Model file for the job. Use its own axes, mm. A direction names the side the tool comes from. Round coordinates to 2 decimals unless told otherwise and drop trailing zeros. Order: outer loops, then holes, each group sorted by start corner. A loop starts at its lowest first (then second) coordinate and runs counter-clockwise, first axis right, second up. Notation, with made-up numbers: (88, -14.5) -> (138, -14.5) arc R16 cw to (138, -4.5) -> close; hole circle Ø4 at (54, 32). An arc over 180 degrees is marked (long way). Use CSV: the item, a comma, the result in double quotes.
```python
from build123d import *

# Parameters (mm, degrees)
F1_DEPTH = 5


with BuildPart() as f1:
    # F0 (on Top) → F1 (new body)
    with BuildSketch(Plane.XY):
        with BuildLine():
            Line((-4.36566, 79.626773), (-32.035204, 75.337673))
            Line((-32.035204, 75.337673), (-22.550609, 14.151324))
            Line((-22.550609, 14.151324), (-13.305154, 10.567361))
            ThreePointArc((-13.305154, 10.567361), (-11.394923, 13.178449), (-8.43507, 14.484602))
            ThreePointArc((-8.43507, 14.484602), (-3.410814, 13.054214), (-1.227681, 8.308365))
            ThreePointArc((-1.227681, 8.308365), (-1.334221, 7.159279), (-1.650209, 6.049369))
            ThreePointArc((-1.650209, 6.049369), (-3.56044, 3.438281), (-6.520293, 2.132127))
            Line((-6.520293, 2.132127), (-5.001368, -7.666653))
            Line((-5.001368, -7.666653), (52.729861, -30.045928))
            Line((52.729861, -30.045928), (62.850163, -3.938851))
            Line((62.850163, -3.938851), (5.118934, 18.440424))
            Line((5.118934, 18.440424), (-4.36566, 79.626773))
        make_face()
        with BuildLine():
            Line((-13.305154, 10.567361), (-22.550609, 14.151324))
            Line((-22.550609, 14.151324), (-70.797245, -24.65575))
            Line((-70.797245, -24.65575), (-53.248003, -46.473727))
            Line((-53.248003, -46.473727), (-5.001368, -7.666653))
            Line((-5.001368, -7.666653), (-6.520293, 2.132127))
            ThreePointArc((-6.520293, 2.132127), (-12.347765, 4.391123), (-13.305154, 10.567361))
        make_face()
    extrude(amount=F1_DEPTH)


solid = f1.part
```
Q1. Cut at B-B (y = -18.5). Give the cut face in (x, z), plus the area to 3 significant figures.
From the geometry:
outline,"(-63.14, 0) -> (-18.47, 0) -> (-18.47, 5) -> (-63.14, 5) -> close; (22.95, 0) -> (57.21, 0) -> (57.21, 5) -> (22.95, 5) -> close"
area,"395 mm²"
Q2. Cut at D-D (y = 49.5). Give the cut face in (x, z), plus the area to 3 significant figures.
From the geometry:
outline,"(-28.03, 0) -> (0.3, 0) -> (0.3, 5) -> (-28.03, 5) -> close"
area,"142 mm²"
Q3. Which spindle directions (+Z, -Z, +X, -X, +Y, -Y) get a long thin tool onto all of the face, cutting with end or side? Do faces 5 (the flat face through (57.719, -17.175, 2.465)), 6 (the flat face through (23.46, -18.7, 2.46)). Say none if no direction does.
From the geometry:
face 5,"+Z, -Z, +X, -Y"
face 6,"+Z, -Z, -Y"
Q4. Probe line 1 along Y through (x, z) = (-44.5, 0.7); line 2 along Y through (x, z) = (-40.5, 3.4); line 3 along X through (y, z) = (74, 3.5). List the from-to ranges inside material, lowest first.
From the geometry:
line 1,"y = -39.44 to -3.5"
line 2,"y = -36.22 to -0.29"
line 3,"x = -31.83 to -3.49"
Q5. Cut at A-A (z = 3.9). Give the cut face in (x, y), plus the area to 3 significant figures.
From the geometry:
outline,"(-70.8, -24.66) -> (-53.25, -46.47) -> (-5, -7.67) -> (52.73, -30.05) -> (62.85, -3.94) -> (5.12, 18.44) -> (-4.37, 79.63) -> (-32.04, 75.34) -> (-22.55, 14.15) -> close; hole (-13.31, 10.57) arc R6.25 ccw to (-6.52, 2.13) arc R6.25 ccw to (-1.65, 6.05) arc R6.25 ccw to (-1.23, 8.31) arc R6.25 ccw to (-8.44, 14.48) arc R6.25 ccw to start"
area,"5,420 mm²"
Q6. Mould opens along Y. For faces 1 (the flat face through (-46.336, -4.981, 2.465)), 2 (the flat face through (-29.46, -27.34, 2.46)), 3 (the flat face through (-14, 3, 0)), 4 (the flat face through (-27.36, 45.17, 2.46)) say: +Y half, -Y half, draft (parallel to the pull), parting line (faces both ways), or undercut.
From the geometry:
face 1,"undercut"
face 2,"-Y half"
face 3,"draft"
face 4,"undercut"
Q7. Cut at C-C (x = 43). Give the cut face in (y, z), plus the area to 3 significant figures.
From the geometry:
outline,"(-26.27, 0) -> (3.76, 0) -> (3.76, 5) -> (-26.27, 5) -> close"
area,"150 mm²"
Q8. Pin check, flat tips, straight feed: pin 1 (2 mm diameter, centred on y = 16.5, z = 2.5, fed in from -X); pin 2 (2 mm diameter, centred on x = 24, z = 3.5, fed in from +Y); pin 3 (2 mm diameter, centred on y = -26, z = 3, fed in from +X). Stop position of each tip, or through.
From the geometry:
pin 1,"stops at x = -23.07"
pin 2,"stops at y = 11.51"
pin 3,"stops at x = 54.69"
